```python
from build123d import *

# Parameters (mm, degrees)
CROQUIS1_W              = 105
CROQUIS1_H              = 50.8
SALIENTE_EXTRUIR1_DEPTH = 12.7
CROQUIS2_W              = 24.650197811
CROQUIS2_H              = 2.575416839
CORTAR_EXTRUIR1_DEPTH   = 109.772468943
CROQUIS3_R              = 2.5
CORTAR_EXTRUIR2_DEPTH   = 60.688357324


with BuildPart() as part:
    # Croquis1 → Saliente-Extruir1 (new body)
    with BuildSketch(Plane(origin=(0, 0, 0), x_dir=(1, 0, 0), z_dir=(0, 1, 0))):
        Rectangle(CROQUIS1_W, CROQUIS1_H)
    extrude(amount=SALIENTE_EXTRUIR1_DEPTH)

    # Croquis2 → Cortar-Extruir1 (cut, through all)
    with BuildSketch(Plane(origin=(52.5, 0, 0), x_dir=(0, 0, -1), z_dir=(1, 0, 0))):
        Polygon((-25.4, 6.35), (-9.701031489, 12.7), (-25.4, 12.7), align=None)
        with Locations((-4.925098905, 1.28770842)):
            Rectangle(CROQUIS2_W, CROQUIS2_H)
        Polygon((25.4, 0), (25.4, 12.7), (7.4, 12.7), (7.4, 2.575416839), (7.4, 0), align=None)
    extrude(amount=-CORTAR_EXTRUIR1_DEPTH, mode=Mode.SUBTRACT)

    # Croquis3 → Cortar-Extruir2 (cut, through all)
    with BuildSketch(Plane(origin=(0, 12.7, 0), x_dir=(1, 0, 0), z_dir=(0, 1, 0))):
        with Locations(Location((0, 0, 0), (0, 0, 270))):
            Circle(CROQUIS3_R)
        with Locations(Location((-40, 0, 0), (0, 0, 270))):
            Circle(CROQUIS3_R)
        with Locations(Location((40, 0, 0), (0, 0, 270))):
            Circle(CROQUIS3_R)
    extrude(amount=-CORTAR_EXTRUIR2_DEPTH, mode=Mode.SUBTRACT)


solid = part.part
```
For this review, take the finished solid that the model builds, in its own axes (mm). A direction names the side the tool comes from. Coordinates: 2 decimals unless noted, no trailing zeros. Loops run counter-clockwise (first coordinate to the right, second up) from the corner with the lowest first, then second, coordinate; pieces in that order, holes last. Notation, with made-up numbers: (-26.75, 51.25) -> (10.25, 51.25) arc R18 ccw to (10.25, 83.25) -> close; hole circle Ø3 at (74.25, 70.25). An arc over 180 degrees is marked (long way). Return JSON: item names as keys, results as strings. Group by question number.
(1) Consider section D-D, the plane y = 11.75. Give the boundary of the cut face in (x, z), plus the area to 3 significant figures.
(2) Consider section A-A, the plane z = 0. Give the boundary of the cut face in (x, y), plus the area to 3 significant figures.
(3) For pin 1 Ø3 at (x, z) = (3.5, 18.5) entering from +Y; pin 2 Ø6 at (x, z) = (-16, 15.5) entering from +Y; pin 3 Ø8 at (x, z) = (0, 0) entering from -Y, all flat-tipped, find the tip position at first contact; note any pin that passes through.
(4) Consider section C-C, the plane y = 4.25. Give the boundary of the cut face in (x, z), plus the area to 3 significant figures.
(5) Mouldability with a two-part tool opening along X and no side actions: class faces 3 (the flat face through (-1, 3, 25.4)), 4 (the flat face through (-52.5, 6, 9)), 5 (the cylindrical face through (-42.44, 7.71, -0.54)) as pulls with the +X half, pulls with the -X half, needs draft (parallel to the pull), parting line crosses it, or undercut.
(6) To check wall thickness, follow L1, parallel to X at y = 4.75, z = 0; L2, parallel to X at y = 8.5, z = 0.5; L3, parallel to Y at x = 10.5, z = 1. State the ranges of each line that lie inside material, in increasing order.
(7) Tool access review of faces 1 (the flat face through (1, 1, 17.25)), 2 (the cylindrical face through (-2.44, 7.71, -0.54)): name each direction out of +Z, -Z, +X, -X, +Y, -Y from which nothing blocks a thin tool from reaching the whole face with its end or side.
(8) Consider section B-B, the plane x = 0. Give the boundary of the cut face in (y, z).
Results below:
{
 "1": {"outline": "(-52.5, -7.4) -> (52.5, -7.4) -> (52.5, 12.05) -> (-52.5, 12.05) -> close; hole circle Ø5 at (-40, 0); hole circle Ø5 at (0, 0); hole circle Ø5 at (40, 0)", "area": "1,980 mm2"},
 "2": {"outline": "(-52.5, 2.58) -> (-42.5, 2.58) -> (-42.5, 12.7) -> (-52.5, 12.7) -> close; (-37.5, 2.58) -> (-2.5, 2.58) -> (-2.5, 12.7) -> (-37.5, 12.7) -> close; (2.5, 2.58) -> (37.5, 2.58) -> (37.5, 12.7) -> (2.5, 12.7) -> close; (42.5, 2.58) -> (52.5, 2.58) -> (52.5, 12.7) -> (42.5, 12.7) -> close", "area": "911 mm2"},
 "3": {"pin 1": "stops at y = 9.75", "pin 2": "stops at y = 11.57", "pin 3": "stops at y = 2.58"},
 "4": {"outline": "(-52.5, -7.4) -> (52.5, -7.4) -> (52.5, 25.4) -> (-52.5, 25.4) -> close; hole circle Ø5 at (-40, 0); hole circle Ø5 at (0, 0); hole circle Ø5 at (40, 0)", "area": "3,390 mm2"},
 "5": {"face 3": "needs draft", "face 4": "pulls with the -X half", "face 5": "undercut"},
 "6": {"L1": "x = -52.5 to -42.5, -37.5 to -2.5, 2.5 to 37.5, 42.5 to 52.5", "L2": "x = -52.5 to -42.45, -37.55 to -2.45, 2.45 to 37.55, 42.45 to 52.5", "L3": "y = 2.58 to 12.7"},
 "7": {"face 1": "-Z, +X, -X, -Y", "face 2": "+Y, -Y"},
 "8": {"outline": "(0, 17.25) -> (2.58, 17.25) -> (2.58, 2.5) -> (12.7, 2.5) -> (12.7, 9.7) -> (6.35, 25.4) -> (0, 25.4) -> close; (2.58, -7.4) -> (12.7, -7.4) -> (12.7, -2.5) -> (2.58, -2.5) -> close"}
}
